The figure shows three views and two pictorial views of one solid part (mm, origin at its lowest corner). Answer the questions. Give positions to 0.01 mm unless a question says otherwise; leave off trailing zeros. Order: outer loops, then holes, each group sorted by start corner. A loop starts at its lowest first (then second) coordinate and runs counter-clockwise, first axis right, second up. Notation, with made-up numbers: (33.25, -30.5) -> (50.25, -30.5) arc R32 cw to (50.25, 0.5) -> close; hole circle Ø11 at (4.5, 20). An arc over 180 degrees is marked (long way). Use one line per item in the form item = value.
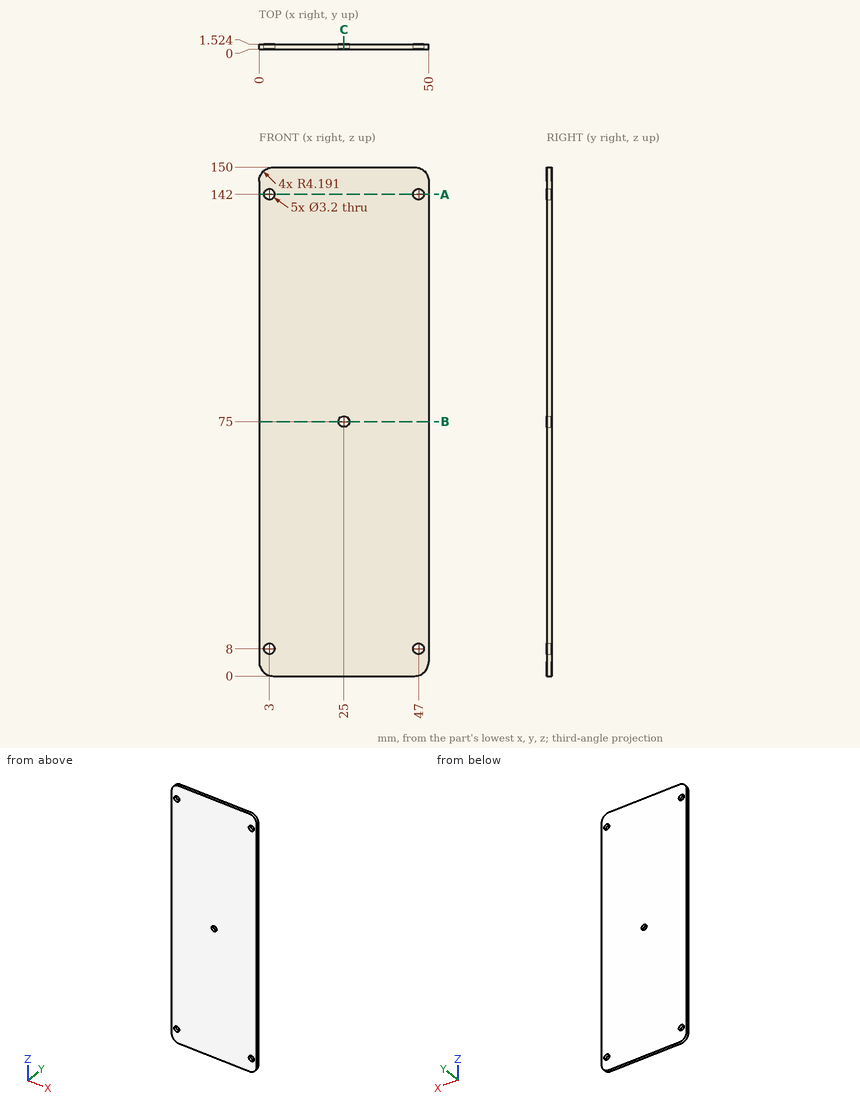
Item 1: The part is cut by section B-B on z = 75. Give the vertices of the cut face in (x, y).
Checks:
outline = (0, 0) -> (23.4, 0) -> (23.4, 1.52) -> (0, 1.52) -> close; (26.6, 0) -> (50, 0) -> (50, 1.52) -> (26.6, 1.52) -> close
Item 2: Straight lines are drawn through the part: L1, parallel to X at y = 0.5, z = 8; L2, parallel to Z at x = 25, y = 0.35; L3, parallel to Z at x = 47, y = 0.7. For each, find the intervals that lie inside material, in ascending order. Write a range as from..to.
Checks:
L1 = 0..1.4, 4.6..45.4, 48.6..50
L2 = 0..73.4, 76.6..150
L3 = 0.17..6.4, 9.6..140.4, 143.6..149.83
Item 3: The part is cut by section C-C on x = 25. Give the vertices of the cut face in (y, z), and give its area (3 significant figures).
Checks:
outline = (0, 0) -> (1.52, 0) -> (1.52, 73.4) -> (0, 73.4) -> close; (0, 76.6) -> (1.52, 76.6) -> (1.52, 150) -> (0, 150) -> close
area = 224 mm²
Item 4: The part is cut by section A-A on z = 142. Give the vertices of the cut face in (x, y), and give its area (3 significant figures).
Checks:
outline = (0, 0) -> (1.4, 0) -> (1.4, 1.52) -> (0, 1.52) -> close; (4.6, 0) -> (45.4, 0) -> (45.4, 1.52) -> (4.6, 1.52) -> close; (48.6, 0) -> (50, 0) -> (50, 1.52) -> (48.6, 1.52) -> close
area = 66.4 mm²
Item 5: Given pin 1 Ø1.9 at (x, z) = (47, 142) entering from +Y, flat-ended and moving along its own axis, determine where the tip first touches the part or whether it passes through.
Checks:
pin_1 = through
